```python
from build123d import *

# Parameters (mm, degrees)
F3_W     = 150
F3_H     = 150
F4_DEPTH = 500
F6_DEPTH = 75
F7_W     = 50
F7_H     = 100
F8_DEPTH = 60


with BuildPart() as f4:
    # F3 (on Front) → F4 (new body, symmetric)
    with BuildSketch(Plane.XZ):
        Rectangle(F3_W, F3_H)
    extrude(amount=F4_DEPTH, both=True)

    # F5 (on Right) → F6 (cut, symmetric)
    with BuildSketch(Plane.YZ):
        Polygon((-500, 75), (-500, 46.1324865405), (-450, 75), align=None)
        Polygon((-213.3974596216, -25), (-300, -75), (0, -75), (300, -75), (213.3974596216, -25), (0, -25), align=None)
        Polygon((450, 75), (500, 46.1324865405), (500, 75), align=None)
    extrude(amount=F6_DEPTH, both=True, mode=Mode.SUBTRACT)

    # F7 (on face) → F8 (cut)
    with BuildSketch(Plane.XY.offset(75)):
        with Locations((0, 400)):
            Rectangle(F7_W, F7_H)
        with Locations((0, -400)):
            Rectangle(F7_W, F7_H)
    extrude(amount=-F8_DEPTH, mode=Mode.SUBTRACT)


solid = f4.part
```
Work out the finished part from the listing and answer in its coordinate system (mm). A direction names the side the tool comes from. Give positions to 0.01 mm unless a question says otherwise; leave off trailing zeros. Write each loop counter-clockwise with the first axis right and the second up, starting at its lowest first coordinate (ties: lowest second). Pieces come first, ordered by that corner, then holes. Notation, with made-up numbers: (41.5, -7.75) -> (70.5, -7.75) arc R21 ccw to (70.5, 5.25) -> close; hole circle Ø7 at (-13, 87.25). An arc over 180 degrees is marked (long way). Write each question's results on one line, items separated by ' | '.
1. Determine the mould class of faces 4 (the flat face through (75, -7, 16)), 5 (the flat face through (-1.05, -475.35, 60.364)), 6 (the flat face through (-25, -401, 45)) for opening direction X: +X half, -X half, draft (parallel to the pull), parting line (faces both ways), or undercut.
Data:
face 4: +X half | face 5: draft | face 6: undercut
2. Straight lines are drawn through the part: L1, parallel to Y at x = 17, z = 22.5; L2, parallel to Y at x = -22, z = 55; L3, parallel to Z at x = 34, y = -67.5. For each, find the intervals that lie inside material, in ascending order.
Data:
L1: -500 to -450, -350 to 350, 450 to 500 | L2: -484.64 to -450, -350 to 350, 450 to 484.64 | L3: -25 to 75
3. A tool of negligible diameter and unlimited length cuts with its end or side. For faces 1 (the flat face through (1.05, 474.65, 60.77)), 2 (the flat face through (25, 399, 45)), 3 (the flat face through (-1, 3, -25)), from which of +Z, -Z, +X, -X, +Y, -Y can it reach the whole face along a straight path? Write none if from no direction.
Data:
face 1: +Z, +X, -X, +Y | face 2: +Z | face 3: -Z, +X, -X
4. Each of these flat-tipped pins is pushed along its axis until it touches: pin 1 Ø25 at (x, y) = (10, -381) entering from +Z; pin 2 Ø15 at (x, z) = (9.5, 59) entering from +Y. Where does it stop, or does it pass through?
Data:
pin 1: z = 15 | pin 2: y = 490.7
5. Find section A-A on z = -50. Determine the outline of the cut face in (x, y), and give its area (3 significant figures).
Data:
outline: (-75, -500) -> (75, -500) -> (75, -256.7) -> (-75, -256.7) -> close; (-75, 256.7) -> (75, 256.7) -> (75, 500) -> (-75, 500) -> close | area: 73,000 mm^2
6. Find section D-D on y = 151.5. Determine the outline of the cut face in (x, z).
Data:
outline: (-75, -25) -> (75, -25) -> (75, 75) -> (-75, 75) -> close
7. Find section B-B on x = -55.5. Determine the outline of the cut face in (y, z), and give its area (3 significant figures).
Data:
outline: (-500, -75) -> (-300, -75) -> (-213.4, -25) -> (213.4, -25) -> (300, -75) -> (500, -75) -> (500, 46.13) -> (450, 75) -> (-450, 75) -> (-500, 46.13) -> close | area: 123,000 mm^2
8. Find section C-C on z = 31. Determine the outline of the cut face in (x, y).
Data:
outline: (-75, -500) -> (75, -500) -> (75, 500) -> (-75, 500) -> close; hole (-25, -450) -> (25, -450) -> (25, -350) -> (-25, -350) -> close; hole (-25, 350) -> (25, 350) -> (25, 450) -> (-25, 450) -> close
